```python
from build123d import *

# Parameters (mm, degrees)
SKETCH_1_R          = 2.5
EXTRUDE_1_DEPTH     = 5
SKETCH_2_W          = 10
SKETCH_2_H          = 5
EXTRUDE_2_DEPTH     = 10
EXTRUDE_3_DEPTH     = 5
CUT_EXTRUDE_1_DEPTH = 43.673176587


with BuildPart() as part:
    # Эскиз1 → Бобышка-Вытянуть1 (new body)
    with BuildSketch(Plane(origin=(0, 0, 0), x_dir=(1, 0, 0), z_dir=(0, 1, 0))):
        with BuildLine():
            Line((3, 0), (7, 0))
            ThreePointArc((7, 0), (9.121320344, 0.878679656), (10, 3))
            Line((10, 3), (10, 30))
            Line((10, 30), (0, 30))
            Line((0, 30), (0, 3))
            ThreePointArc((0, 3), (0.878679656, 0.878679656), (3, 0))
        make_face()
        with Locations(Location((5, 8.25, 0), (0, 0, 270))):
            Circle(SKETCH_1_R, mode=Mode.SUBTRACT)
    extrude(amount=EXTRUDE_1_DEPTH)

    # Эскиз2 → Бобышка-Вытянуть2 (add)
    with BuildSketch(Plane(origin=(0, 0, -30), x_dir=(-1, 0, 0), z_dir=(0, 0, -1))):
        with Locations((-5, 2.5)):
            Rectangle(SKETCH_2_W, SKETCH_2_H)
    extrude(amount=EXTRUDE_2_DEPTH)

    # Эскиз4 → Бобышка-Вытянуть3 (add)
    with BuildSketch(Plane(origin=(0, 5, 0), x_dir=(1, 0, 0), z_dir=(0, 1, 0))):
        with BuildLine():
            Line((13, 40), (10, 40))
            Line((10, 40), (10, 29))
            ThreePointArc((10, 29), (10.292893219, 29.707106781), (11, 30))
            Line((11, 30), (13, 30))
            ThreePointArc((13, 30), (13.707106781, 30.292893219), (14, 31))
            Line((14, 31), (14, 39))
            ThreePointArc((14, 39), (13.707106781, 39.707106781), (13, 40))
        make_face()
    extrude(amount=-EXTRUDE_3_DEPTH)

    # Эскиз5 → Вырез-Вытянуть1 (cut, through all)
    with BuildSketch(Plane(origin=(0, 5, 0), x_dir=(1, 0, 0), z_dir=(0, 1, 0))):
        with BuildLine():
            Line((0, 38.89263227), (0, 39))
            ThreePointArc((0, 39), (0.292893219, 39.707106781), (1, 40))
            Line((1, 40), (1.042017626, 40))
            Line((1.042017626, 40), (0.948883757, 40.294542088))
            Line((0.948883757, 40.294542088), (-0.497142104, 40.245524262))
            Line((-0.497142104, 40.245524262), (-0.497142104, 39.412221223))
            Line((-0.497142104, 39.412221223), (0, 38.89263227))
        make_face()
    extrude(amount=-CUT_EXTRUDE_1_DEPTH, mode=Mode.SUBTRACT)


solid = part.part
```
CAD build for the part. Positions are in the model's coordinates, mm. A direction names the side the tool comes from. Coordinates: 2 decimals unless noted, no trailing zeros. Order: outer loops, then holes, each group sorted by start corner. A loop starts at its lowest first (then second) coordinate and runs counter-clockwise, first axis right, second up. Notation, with made-up numbers: M 64.5,85.5 L 88.5,85.5 A24 cw 88.5,120.5 Z; hole C -24,-10 d10. An arc over 180 degrees is marked long. Answer as CSV lines item,"result".
1) Cut at A-A (z = -8.25). List the corners of the cut face in (x, y), then the cut area to 3 significant figures.
Verdict:
outline,"M 0,0 L 2.5,0 L 2.5,5 L 0,5 Z; M 7.5,0 L 10,0 L 10,5 L 7.5,5 Z"
area,"25.0 mm2"
2) Flat gauge pin, fed straight in: P1, Ø2, axis at x = 12.5, y = 2.5, coming from the +Z side. Where does the tip first touch, or does it go through?
Verdict:
P1,"z = -30"
3) Cut at B-B (y = 4.55). List the corners of the cut face in (x, z), then the cut area to 3 significant figures.
Verdict:
outline,"M 0,-39 A1 ccw 1,-40 L 13,-40 A1 ccw 14,-39 L 14,-31 A1 ccw 13,-30 L 11,-30 A1 cw 10,-29 L 10,-3 A3 ccw 7,0 L 3,0 A3 ccw 0,-3 Z; hole C 5,-8.25 d5"
area,"416 mm2"
4) Mould opens along Z. For faces 3 (the flat face through (12, 3, -30)), 4 (the cylindrical face through (13.715, 2.535, -39.699)), 5 (the cylindrical face through (6.69, 2.46, -10.09)) say: released by +Z, released by -Z, zero draft, split by the parting line, or undercut.
Verdict:
face 3,"released by +Z"
face 4,"released by -Z"
face 5,"undercut"
5) Cut at C-C (x = 3.5). List the corners of the cut face in (y, z), then the cut area to 3 significant figures.
Verdict:
outline,"M 0,-40 L 5,-40 L 5,-10.25 L 0,-10.25 Z; M 0,-6.25 L 5,-6.25 L 5,0 L 0,0 Z"
area,"180 mm2"
6) 3-axis set-ups, long thin cutter, end or side, ignore diameter. For faces 1 (the flat face through (10, 2, -16)), 2 (the cylindrical face through (0.86, 2.46, -0.9)): which of +Z, -Z, +X, -X, +Y, -Y reach the whole face in a straight line?
Verdict:
face 1,"+Z, +X, +Y, -Y"
face 2,"+Z, -X, +Y, -Y"
7) Drill centre lines: L1, parallel to X at y = 2.15, z = -8.25; L2, parallel to Z at x = 6.75, y = 1; L3, parallel to X at y = 0.7, z = -3.5. Where is each one in solid material? Low to high. Write a range as from..to.
Verdict:
L1,"0..2.5, 7.5..10"
L2,"-40..-10.04, -6.46..0"
L3,"0..10"
8) Cut at D-D (z = -21.5). List the corners of the cut face in (x, y), then the cut area to 3 significant figures.
Verdict:
outline,"M 0,0 L 10,0 L 10,5 L 0,5 Z"
area,"50.0 mm2"
